Design review of the part built by this model. Coordinates are the model's own, in mm. A direction names the side the tool comes from. Round coordinates to 2 decimals unless told otherwise and drop trailing zeros. Loops run counter-clockwise (first coordinate to the right, second up) from the corner with the lowest first, then second, coordinate; pieces in that order, holes last. Notation, with made-up numbers: M -4,18.5 L 41,18.5 A34 ccw 41,52.5 Z; hole C 66,26.5 d8. An arc over 180 degrees is marked long. One line per item, written item: value. Start each with the question number.
Item 1: For line 1 along Z through (x, y) = (-67.5, 3.5); line 2 along Z through (x, y) = (-66, 1.25); line 3 along Y through (x, z) = (24, -29.5), list the stretches that pass through material, from the lowest coordinate up.
Item 2: We need section B-B (x = -59). Write out the cut boundary in (y, z).
Item 3: We need section A-A (x = 53). Write out the cut boundary in (y, z).
Item 4: Clearance check with flat-ended pins moving along their axes: pin 1 (1.5 mm diameter, centred on y = 2.5, z = -9.5, fed in from +X); pin 2 (1.6 mm diameter, centred on y = 2.5, z = 31.5, fed in from -X); pin 3 (4 mm diameter, centred on x = 33.69, z = 52.86, fed in from -Y); pin 4 (1.5 mm diameter, centred on x = -48.5, z = -31, fed in from +Y). State where each tip first meets the part, or that it passes through.
Item 5: Mouldability with a two-part tool opening along Z and no side actions: class faces 1 (the cylindrical face through (-97.88, 2.03, 63.36)), 2 (the cylindrical face through (-80.733, 2.028, 48.359)), 3 (the flat face through (65.693, 2, 57)) as released by +Z, released by -Z, zero draft, split by the parting line, or undercut.
Item 6: For faces 4 (the flat face through (59, 2.4, -51)), 5 (the flat face through (-94, 3, -53)), 6 (the cylindrical face through (-97.8, 2.03, -46.56)), list the 3-axis set-ups (+Z, -Z, +X, -X, +Y, -Y) from which the entire face can be reached by the end or side of a thin tool; tool diameter is ignored.
from build123d import *

# Parameters (mm, degrees)
BOSS_EXTRUDE1_DEPTH = 4
SKETCH2_R           = 1.55
CUT_EXTRUDE3_DEPTH  = 119.680122062
FILLET1_R           = 5
SKETCH5_R           = 1.525
CUT_EXTRUDE4_DEPTH  = 10
SKETCH5_3_R         = 4.5
CUT_EXTRUDE5_DEPTH  = 1
CUT_EXTRUDE6_DEPTH  = 2.4
SKETCH8_W           = 25
SKETCH8_H           = 125
BOSS_EXTRUDE4_DEPTH = 5
CUT_EXTRUDE7_DEPTH  = 160.724398205
FILLET5_R           = 5
SKETCH10_W          = 5
SKETCH10_H          = 5.5
CUT_EXTRUDE8_DEPTH  = 5
FILLET7_R           = 1


with BuildPart() as part:
    # Sketch1 → Boss-Extrude1 (new body)
    with BuildSketch(Plane(origin=(0, 0, 0), x_dir=(1, 0, 0), z_dir=(0, 1, 0))):
        Polygon((-79.307015775, 45.137931034), (-79.307015775, -49.862068966), (-99.307015775, -49.862068966), (-99.307015775, -64.862068966), (-68.307015775, -64.862068966), (45.692984225, -64.862068966), (65.692984225, -64.862068966), (65.692984225, -49.862068966), (45.692984225, -49.862068966), (45.692984225, 45.137931034), (65.692984225, 45.137931034), (65.692984225, 60.137931034), (45.692984225, 60.137931034), (-68.307015775, 60.137931034), (-99.307015775, 60.137931034), (-99.307015775, 45.137931034), align=None)
    extrude(amount=BOSS_EXTRUDE1_DEPTH)

    # Sketch2 → Cut-Extrude3 (cut, through all)
    with BuildSketch(Plane(origin=(0, 4, 0), x_dir=(1, 0, 0), z_dir=(0, 1, 0))):
        with Locations(Location((33.692984225, 48.137931034, 0), (0, 0, 270))):
            Circle(SKETCH2_R)
        with Locations(Location((-67.307015775, 48.137931034, 0), (0, 0, 270))):
            Circle(SKETCH2_R)
        with Locations(Location((-67.307015775, -52.862068966, 0), (0, 0, 270))):
            Circle(SKETCH2_R)
        with Locations(Location((33.692984225, -52.862068966, 0), (0, 0, 270))):
            Circle(SKETCH2_R)
    extrude(amount=-CUT_EXTRUDE3_DEPTH, mode=Mode.SUBTRACT)

    # Fillet1
    fillet1_edges = [part.edges().sort_by_distance(p)[0] for p in [
        (65.692984225, 2, -60.137931034),
        (65.692984225, 2, -45.137931034),
        (45.692984225, 2, -45.137931034),
        (45.692984225, 2, 49.862068966),
        (65.692984225, 2, 49.862068966),
        (65.692984225, 2, 64.862068966),
        (-99.307015775, 2, 64.862068966),
        (-99.307015775, 2, 49.862068966),
        (-79.307015775, 2, 49.862068966),
        (-79.307015775, 2, -45.137931034),
        (-99.307015775, 2, -45.137931034),
        (-99.307015775, 2, -60.137931034),
    ]]
    fillet(fillet1_edges, radius=FILLET1_R)

    # Sketch5 → Cut-Extrude4 (cut)
    with BuildSketch(Plane(origin=(0, 4, 0), x_dir=(1, 0, 0), z_dir=(0, 1, 0))):
        with Locations(Location((-91.807015775, 52.637931034, 0), (0, 0, 270))):
            Circle(SKETCH5_R)
        with Locations(Location((-91.807015775, -57.362068966, 0), (0, 0, 270))):
            Circle(SKETCH5_R)
        with Locations(Location((58.192984225, -57.362068966, 0), (0, 0, 270))):
            Circle(SKETCH5_R)
        with Locations(Location((58.192984225, 52.637931034, 0), (0, 0, 270))):
            Circle(SKETCH5_R)
    extrude(amount=-CUT_EXTRUDE4_DEPTH, mode=Mode.SUBTRACT)

    # Sketch5<3> → Cut-Extrude5 (cut)
    with BuildSketch(Plane(origin=(0, 4, 0), x_dir=(1, 0, 0), z_dir=(0, 1, 0))):
        with Locations(Location((-91.807015775, 52.637931034, 0), (0, 0, 270))):
            Circle(SKETCH5_3_R)
    extrude(amount=-CUT_EXTRUDE5_DEPTH, mode=Mode.SUBTRACT)

    # Sketch6 → Cut-Extrude6 (cut)
    with BuildSketch(Plane.XZ):
        Polygon((-88.636873981, 56.89548456), (-89.81787093, 59.87420009), (-92.988012724, 60.340784495), (-94.977157568, 57.828653371), (-93.79616062, 54.849937841), (-90.626018826, 54.383353436), align=None)
        Polygon((61.375334539, 56.987707532), (60.108365894, 59.930884464), (56.92601558, 60.305245897), (55.010633912, 57.736430399), (56.277602557, 54.793253467), (59.459952871, 54.418892034), align=None)
        Polygon((60.682419613, -50.620454529), (57.690516013, -49.473278495), (55.201080626, -51.490755001), (55.703548838, -54.65540754), (58.695452437, -55.802583574), (61.184887825, -53.785107068), align=None)
        Polygon((-88.740685409, -51.707813788), (-91.079355756, -49.517352419), (-94.145686121, -50.447469665), (-94.87334614, -53.568048281), (-92.534675794, -55.75850965), (-89.468345428, -54.828392404), align=None)
    extrude(amount=-CUT_EXTRUDE6_DEPTH, mode=Mode.SUBTRACT)

    # Sketch8 → Boss-Extrude4 (add)
    with BuildSketch(Plane.XZ):
        with Locations((-16.807015775, 2.362068966)):
            Rectangle(SKETCH8_W, SKETCH8_H)
    extrude(amount=BOSS_EXTRUDE4_DEPTH)

    # Sketch9 → Cut-Extrude7 (cut, through all)
    with BuildSketch(Plane.XY.offset(64.862068966)):
        with BuildLine():
            Line((-4.307015775, -5), (-29.307015775, -5))
            add(Edge.make_bspline(
                [(-4.307015775, -5), (-15.592681682, 2.270069745), (-29.307015775, -5)],
                knots=[0, 0, 0, 1, 1, 1], degree=2))
        make_face()
    extrude(amount=-CUT_EXTRUDE7_DEPTH, mode=Mode.SUBTRACT)

    # Fillet5
    fillet5_edges = [part.edges().sort_by_distance(p)[0] for p in [
        (-29.307015775, 0, 2.362068966),
        (-4.307015775, 0, 2.362068966),
    ]]
    fillet(fillet5_edges, radius=FILLET5_R - 0.0001)  # a hair under: the kernel refuses the full size

    # Sketch10 → Cut-Extrude8 (cut)
    with BuildSketch(Plane.XZ):
        with Locations((18.192984225, -32.387931034)):
            Rectangle(SKETCH10_W, SKETCH10_H)
        with Locations((18.192984225, 32.112068966)):
            Rectangle(SKETCH10_W, SKETCH10_H)
        with Locations((-51.807015775, 32.112068966)):
            Rectangle(SKETCH10_W, SKETCH10_H)
        with Locations((-51.807015775, -32.387931034)):
            Rectangle(SKETCH10_W, SKETCH10_H)
    extrude(amount=-CUT_EXTRUDE8_DEPTH, mode=Mode.SUBTRACT)

    # Fillet7
    fillet7_edges = [part.edges().sort_by_distance(p)[0] for p in [
        (20.692984225, 4, -32.387931034),
        (15.692984225, 4, -32.387931034),
        (20.692984225, 0, -32.387931034),
        (15.692984225, 0, -32.387931034),
        (-54.307015775, 4, -32.387931034),
        (-49.307015775, 4, -32.387931034),
        (-54.307015775, 4, 32.112068966),
        (-49.307015775, 4, 32.112068966),
        (20.692984225, 4, 32.112068966),
        (15.692984225, 4, 32.112068966),
        (20.692984225, 0, 32.112068966),
        (15.692984225, 0, 32.112068966),
        (-49.307015775, 0, 32.112068966),
        (-54.307015775, 0, 32.112068966),
        (-49.307015775, 0, -32.387931034),
        (-54.307015775, 0, -32.387931034),
    ]]
    fillet(fillet7_edges, radius=FILLET7_R)


solid = part.part
A:
1. line 1: -60.14 to -49.68, -46.6 to 51.32, 54.4 to 64.86
1. line 2: -60.14 to -48.97, -47.3 to 52.03, 53.7 to 64.86
1. line 3: 0 to 4
2. outline: M 0,-60.14 L 4,-60.14 L 4,64.86 L 0,64.86 Z
3. outline: M 0,-60.14 L 4,-60.14 L 4,-45.14 L 0,-45.14 Z; M 0,49.86 L 4,49.86 L 4,64.86 L 0,64.86 Z
4. pin 1: x = 45.69
4. pin 2: x = -79.31
4. pin 3: y = 0
4. pin 4: y = 4
5. face 1: released by +Z
5. face 2: undercut
5. face 3: zero draft
6. face 4: -Y
6. face 5: +Y
6. face 6: -X, +Y, -Y
